Read the model definition and answer for the solid it produces. Units are mm, in the model's axes. Give positions to 0.01 mm unless a question says otherwise; leave off trailing zeros. Loops run counter-clockwise (first coordinate to the right, second up) from the corner with the lowest first, then second, coordinate; pieces in that order, holes last. Notation, with made-up numbers: (35.5, 28.25) - (40.5, 28.25) arc R26 cw to (40.5, 43.25) - close; hole circle Ø6 at (-25.5, 66). An arc over 180 degrees is marked (long way). Put each result on its own line as item: value. Start each with the question number.
1. Consider L1, parallel to Y at x = -33.5, z = 2.8; L2, parallel to X at y = -18.5, z = 1.4 (3 decimals); L3, parallel to X at y = 63.5, z = 2.9 (1 decimal). Determine where each line is inside the solid, lowest interval first. Write a range as from..to.
2. A cutting plane is placed at A-A, the plane y = -19.05. Determine the outline of the cut face in (x, z) (3 decimals).
3. A cutting plane is placed at B-B, the plane x = 0. Determine the outline of the cut face in (y, z) (3 decimals).
4. Given pin 1 Ø5.5 at (x, y) = (-61.71, 37.9) entering from +Z, flat-ended and moving along its own axis, determine where the tip first touches the part or whether it passes through.
5. A cutting plane is placed at C-C, the plane z = 1.5. Count the separate pieces of the cut face and the enclosed holes in it, plus the area to 3 significant figures.
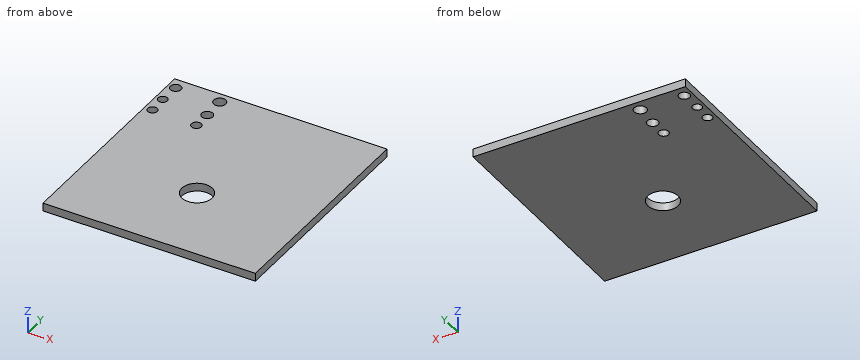
```python
from build123d import *

# Parameters (mm, degrees)
F0_W     = 133.35
F0_H     = 139.7
F1_DEPTH = 5.08
F2_R     = 9.525
F3_DEPTH = 27.178
F4_R     = 3.381666
F4_R_2   = 2.993363
F4_R_3   = 2.952318
F4_R_4   = 3.849352
F4_R_5   = 3.508168
F4_R_6   = 3.090783
F5_DEPTH = 25.4


with BuildPart() as f1:
    # F0 (on Top) → F1 (new body)
    with BuildSketch(Plane.XY):
        Rectangle(F0_W, F0_H)
    extrude(amount=F1_DEPTH)

    # F2 (on Top) → F3 (cut)
    with BuildSketch(Plane.XY):
        with Locations((0, -19.05)):
            Circle(F2_R)
    extrude(amount=F3_DEPTH, mode=Mode.SUBTRACT)

    # F4 (on face) → F5 (cut)
    with BuildSketch(Plane.XY.offset(5.08)):
        with Locations((-61.71133, 62.55158)):
            Circle(F4_R)
        with Locations((-61.71133, 37.904385)):
            Circle(F4_R_2)
        with Locations((-62.084772, 49.481098)):
            Circle(F4_R_3)
        with Locations((-34.263328, 62.925018)):
            Circle(F4_R_4)
        with Locations((-33.703163, 48.734214)):
            Circle(F4_R_5)
        with Locations((-33.703163, 37.157502)):
            Circle(F4_R_6)
    extrude(amount=-F5_DEPTH, mode=Mode.SUBTRACT)


solid = f1.part
```
Return value:
1. L1: y = -69.85..34.07, 40.24..45.23, 52.24..59.15, 66.7..69.85
1. L2: x = -66.675..-9.509, 9.509..66.675
1. L3: x = -66.7..-65, -58.5..-38.1, -30.5..66.7
2. outline: (-66.675, 0) - (-9.525, 0) - (-9.525, 5.08) - (-66.675, 5.08) - close; (9.525, 0) - (66.675, 0) - (66.675, 5.08) - (9.525, 5.08) - close
3. outline: (-69.85, 0) - (-28.575, 0) - (-28.575, 5.08) - (-69.85, 5.08) - close; (-9.525, 0) - (69.85, 0) - (69.85, 5.08) - (-9.525, 5.08) - close
4. pin 1: passes through
5. separate pieces: 1
5. enclosed holes: 7
5. area: 18,100 mm2
